The model under review builds one solid part; all positions refer to its coordinate system, in mm. Coordinates: 2 decimals unless noted, no trailing zeros. Write each loop counter-clockwise with the first axis right and the second up, starting at its lowest first coordinate (ties: lowest second). Pieces come first, ordered by that corner, then holes.
1) Add section C-C, the plane y = 73.5. State the section outline as (x, z) points.
2) Add section B-B, the plane z = 25. State the section outline as (x, y) points.
3) Add section A-A, the plane x = 14.5. State the section outline as (y, z) points, then the cut area to 3 significant figures.
4) For line 1 (Z direction, x = 2.75, y = 54.5); line 2 (Z direction, x = 15.25, y = 24.5); line 3 (Y direction, x = 18.25, z = 4), list the stretches that pass through material, from the lowest coordinate up.
5) For P1, Ø12, axis at x = 10.5, z = 13, coming from the +Y side; P2, Ø6, axis at y = 8, z = -20, coming from the -X side; P3, Ø1.5, axis at x = 5.5, y = -1.5, coming from the +Z side, all flat-tipped, find the tip position at first contact; note any pin that passes through.
from build123d import *

# Parameters (mm, degrees)
F1_DEPTH = 25.4


with BuildPart() as f1:
    # F0 (on Right) → F1 (new body)
    with BuildSketch(Plane.YZ):
        with BuildLine():
            ThreePointArc((88.932255, 0), (86.601213, 7.333124), (80.463797, 11.974308))
            ThreePointArc((80.463797, 11.974308), (63.532255, 0), (80.463797, -11.974308))
            ThreePointArc((80.463797, -11.974308), (86.601213, -7.333124), (88.932255, 0))
        make_face()
        with BuildLine():
            ThreePointArc((12.694627, 35.922924), (31.106874, 21.999372), (38.1, 0))
            ThreePointArc((38.1, 0), (31.106874, -21.999372), (12.694627, -35.922924))
            Line((12.694627, -35.922924), (80.463797, -11.974308))
            ThreePointArc((80.463797, -11.974308), (63.532255, 0), (80.463797, 11.974308))
            Line((80.463797, 11.974308), (12.694627, 35.922924))
        make_face()
        with BuildLine():
            ThreePointArc((12.694627, -35.922924), (31.106874, -21.999372), (38.1, 0))
            ThreePointArc((38.1, 0), (31.106874, 21.999372), (12.694627, 35.922924))
            ThreePointArc((12.694627, 35.922924), (-38.1, 0), (12.694627, -35.922924))
        make_face()
    extrude(amount=F1_DEPTH)


solid = f1.part
Geometry results:
1. outline: (0, -14.44) - (25.4, -14.44) - (25.4, 14.44) - (0, 14.44) - close
2. outline: (0, -28.75) - (25.4, -28.75) - (25.4, 43.6) - (0, 43.6) - close
3. outline: (12.69, -35.92) - (80.46, -11.97) arc R12.7 ccw to (80.46, 11.97) - (12.69, 35.92) arc R38.1 ccw (long way) to start
3. area: 6,620 mm2
4. line 1: z = -21.15 to 21.15
4. line 2: z = -31.75 to 31.75
4. line 3: y = -37.89 to 88.29
5. P1: stops at y = 86.83
5. P2: stops at x = 0
5. P3: stops at z = 38.09
